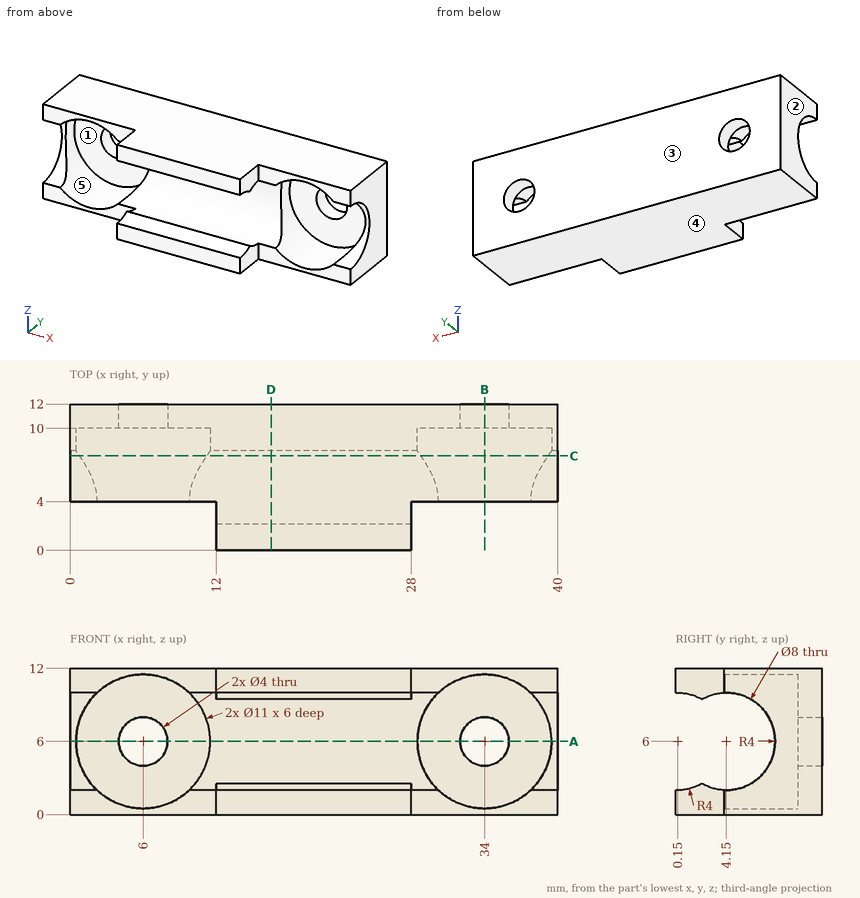
The drawing under review shows one solid part. Ordinate dimensions are in mm from its lowest x, y, z. A direction names the side the tool comes from. Coordinates: 2 decimals unless noted, no trailing zeros. Write each loop counter-clockwise with the first axis right and the second up, starting at its lowest first coordinate (ties: lowest second). Pieces come first, ordered by that corner, then holes. Notation, with made-up numbers: (-21, -34.75) - (-1, -34.75) arc R15 cw to (-1, -14.75) - close; hole circle Ø6 at (69.25, 40.5). An arc over 180 degrees is marked (long way). Use one line per item in the form item = value.
Q1. Consider section B-B (x = 34). Write out the cut boundary in (y, z).
Taken from the geometry:
outline = (4, 0) - (12, 0) - (12, 4) - (10, 4) - (10, 0.5) - (4, 0.5) - close; (4, 11.5) - (10, 11.5) - (10, 8) - (12, 8) - (12, 12) - (4, 12) - close
Q2. Consider section C-C (y = 7.75). Write out the cut boundary in (x, z), plus the area to 3 significant figures.
Taken from the geometry:
outline = (0, 0) - (40, 0) - (40, 4.26) - (39.22, 4.26) arc R5.5 cw to (28.78, 4.26) - (11.22, 4.26) arc R5.5 cw to (0.78, 4.26) - (0, 4.26) - close; (0, 7.74) - (0.78, 7.74) arc R5.5 cw to (11.22, 7.74) - (28.78, 7.74) arc R5.5 cw to (39.22, 7.74) - (40, 7.74) - (40, 12) - (0, 12) - close
area = 226 mm^2
Q3. Insertion check: pin 1 Ø2 at (x, z) = (6, 11) entering from -Y; pin 2 Ø0.6 at (x, z) = (4, 1.5) entering from -Y; pin 3 Ø1.3 at (y, z) = (1, 10.5) entering from +X. Each pin has a flat end and moves straight along its axis. Give the tip position at first contact, or say it passes through.
Taken from the geometry:
pin_1 = 4
pin_2 = 10
pin_3 = 28
Q4. Consider section D-D (x = 16.5). Write out the cut boundary in (y, z), plus the area to 3 significant figures.
Taken from the geometry:
outline = (0, 0) - (12, 0) - (12, 12) - (0, 12) - (0, 10) arc R4 cw to (2.15, 9.46) arc R4 cw (long way) to (2.15, 2.54) arc R4 cw to (0, 2) - close
area = 87.1 mm^2
Q5. Machinability: for the marked faces 4 and 5, which of the approach directions +Z, -Z, +X, -X, +Y, -Y give a long, thin tool a straight path to every point of the face, cutting with its end or side? Answer none if there is none.
Taken from the geometry:
face_4 = -Z, +X, -X, +Y, -Y
face_5 = -Y
Q6. The part is to be moulded in two halves that separate along X. For the marked faces 1, 2 and 3, say which applies: +X half, -X half, draft (parallel to the pull), parting line (faces both ways), or undercut.
Taken from the geometry:
face_1 = undercut
face_2 = -X half
face_3 = draft
Q7. Consider section A-A (z = 6). Write out the cut boundary in (x, y).
Taken from the geometry:
outline = (0, 8.15) - (0.5, 8.15) - (0.5, 10) - (4, 10) - (4, 12) - (0, 12) - close; (8, 10) - (11.5, 10) - (11.5, 8.15) - (28.5, 8.15) - (28.5, 10) - (32, 10) - (32, 12) - (8, 12) - close; (36, 10) - (39.5, 10) - (39.5, 8.15) - (40, 8.15) - (40, 12) - (36, 12) - close
Q8. For probe 1 along X at (y, z) = (7.5, 10); probe 2 along Z at (x, y) = (15.5, 4.15); probe 3 along Z at (x, y) = (6, 10.55), list the stretches that pass through material, from the lowest coordinate up.
Taken from the geometry:
probe_1 = 0 to 2.23, 9.77 to 30.23, 37.77 to 40
probe_2 = 0 to 2, 10 to 12
probe_3 = 0 to 4, 8 to 12
